Autodesk Inventor part; units mm, degrees
ref_plane "YZ Plane" through (0, 0, 0) normal (1, 0, 0) x (0, 1, 0)
ref_plane "XZ Plane" through (0, 0, 0) normal (0, 1, 0) x (-1, 0, 0)
ref_plane "XY Plane" through (0, 0, 0) normal (0, 0, 1) x (1, 0, 0)
sketch "Sketch1" plane through (0, 0, 0) normal (0, 0, 1) x (1, 0, 0)
  line L0 (0, 0) -> (0, 60)
  line L1 (0, 60) -> (80, 60)
  line L2 (80, 60) -> (80, 170)
  line L3 (80, 170) -> (280, 170)
  line L4 (280, 170) -> (280, 0)
  line L5 (0, 0) -> (35, 0)
  line L6 (35, 0) -> (35, 20)
  arc A0 (75, 20) -> (35, 20) centre (55, 20) ccw
  line L7 (75, 20) -> (75, 0)
  line L8 (140, 0) -> (140, 170) construction
  line L9 (75, 0) -> (140, 0)
  line L10 (280, 0) -> (245, 0)
  line L11 (245, 0) -> (245, 20)
  arc A1 (245, 20) -> (205, 20) centre (225, 20) ccw
  line L12 (205, 20) -> (205, 0)
  line L13 (205, 0) -> (140, 0)
  line L14 (145, 170) -> (215, 170)
  line L15 (215, 170) -> (215, 175)
  line L16 (215, 175) -> (145, 175)
  line L17 (145, 175) -> (145, 170)
  line L18 (280, 80) -> (275, 80)
  line L19 (275, 80) -> (275, 130)
  line L20 (275, 130) -> (280, 130)
  line L21 (280, 130) -> (280, 80)
  line L22 (10, 20) -> (15, 20)
  line L23 (15, 20) -> (15, 60)
  line L24 (15, 60) -> (10, 60)
  line L25 (10, 60) -> (10, 20)
  line L26 (20, 60) -> (60, 60)
  line L27 (60, 60) -> (60, 65)
  line L28 (60, 65) -> (20, 65)
  line L29 (20, 65) -> (20, 60)
  line L30 (160, 0) -> (160, -5)
  line L31 (160, -5) -> (120, -5)
  line L32 (120, -5) -> (120, 0)
  dimension "d0" = 60
  dimension "d2" = 110
  dimension "d5" = 20
  dimension "d6" = 40
  dimension "d7" = 70
  dimension "d8" = 5
  dimension "d9" = 5
  dimension "d10" = 50
  dimension "d13" = 5
  dimension "d14" = 40
  dimension "d17" = 40
  dimension "d18" = 5
  dimension "d19" = 40
  dimension "d20" = 5
  dimension "d21" = 20
  dimension "d22" = 0
  dimension "d23" = 170
  dimension "d27" = 35
  dimension "d28" = 80
extrude "Extrusion1" add sketch "Sketch1" along normal blind 5 contours L0 L1 L25 L22 L23 L2 L3 L4 L20 L19 L18 L10 L11 A1 L12 L13 L9 L7 A0 L6 L5 | L1 L23 L22 L25 | L29 L28 L27 L1 | L9 L13 L30 L31 L32 | L17 L16 L15 L3
sketch "Sketch2" plane through (0, 0, 5) normal (0, 0, 1) x (1, 0, 0)
  line L0 (215, 175) -> (145, 175)
  line L1 (145, 175) -> (145, 170)
  line L2 (120, -5) -> (160, -5)
  line L3 (160, -5) -> (160, 0)
  line L4 (0, 60) -> (0, 0)
  line L5 (20, 60) -> (0, 60)
  point P0 (175, 155)
  point P1 (185, 155)
  point P2 (135, 15)
  point P3 (145, 15)
  point P4 (20, 35)
  point P5 (20, 25)
  dimension "d43" = 10
  dimension "d44" = 20
  dimension "d45" = 20
  dimension "d46" = 30
  dimension "d47" = 20
  dimension "d48" = 20
  dimension "d49" = 10
  dimension "d50" = 15
  dimension "d51" = 10
  dimension "d52" = 20
  dimension "d53" = 20
  dimension "d54" = 25
hole "Hole1" at (175, 155, 5) at (185, 155, 5) at (135, 15, 5) at (145, 15, 5) at (20, 35, 5) at (20, 25, 5) direction (0, 0, -1) diameter 4 end through all
sketch "Sketch4" plane through (0, 0, 5) normal (0, 0, 1) x (1, 0, 0)
  line L0 (80, 170) -> (80, 60)
  line L1 (80, 60) -> (60, 60)
  point P0 (0, 0)
  point P1 (95, 80)
  point P2 (95, 90)
  dimension "d63" = 15
  dimension "d64" = 15
  dimension "d65" = 10
  dimension "d66" = 20
hole "Hole3" at (95, 80, 5) at (95, 90, 5) direction (0, 0, -1) diameter 4 end through all
properties part number "side"
Model file for the job. Use its own axes, mm. A direction names the side the tool comes from. Coordinates: 2 decimals unless noted, no trailing zeros. Loops run counter-clockwise (first coordinate to the right, second up) from the corner with the lowest first, then second, coordinate; pieces in that order, holes last. Notation, with made-up numbers: (62.25, -32) -> (72.25, -32) arc R4 cw to (72.25, -25) -> close; hole circle Ø2 at (16, 31.5). An arc over 180 degrees is marked (long way). Use one line per item in the form item = value. Start each with the question number.
(1) Cut at B-B on z = 3.1. Give the number of separate pieces and of enclosed holes in the cut face, and give its area (3 significant figures).
(2) Pull direction X, two halves, no side cores. Call faces 4 (the flat face through (10, 60, 2)), 5 (the flat face through (35, 10, 2)), 6 (the flat face through (20, 63, 2)): pulls with the +X half, pulls with the -X half, needs draft (parallel to the pull), parting line crosses it, or undercut.
(3) Cut at A-A on y = 140.5. Give the cut face in (x, z), and give its area (3 significant figures).
(4) Cut at C-C on x = 109. Give the cut face in (y, z).
(5) Tool access for faces 1 (the flat face through (70, 60, 2)), 2 (the flat face through (40, 65, 2)), 3 (the flat face through (205, 10, 2)): list every direction of +Z, -Z, +X, -X, +Y, -Y with a clear straight run to the whole face (end or side of a thin tool).
(6) Flat gauge pins, fed straight in: pin 1 (2.5 mm diameter, centred on x = 175, y = 155, fed in from +Z); pin 2 (2.5 mm diameter, centred on x = 121, z = 2, fed in from +Y); pin 3 (1.5 mm diameter, centred on x = 65.5, z = 3.5, fed in from +Y); pin 4 (3 mm diameter, centred on y = 124, z = 2, fed in from -X). Where does each tip first touch, or does it go through?
(7) Probe probe 1 along X at (y, z) = (155, 2); probe 2 along X at (y, z) = (15, 2.1); probe 3 along Y at (x, z) = (20.5, 2.6). List the from-to ranges inside material, lowest first. Write a range as from..to.
Values:
q1.separate_pieces = 1
q1.enclosed_holes = 8
q1.area = 36,300 mm2
q2.face_4 = needs draft
q2.face_5 = undercut
q2.face_6 = pulls with the -X half
q3.outline = (80, 0) -> (280, 0) -> (280, 5) -> (80, 5) -> close
q3.area = 1,000 mm2
q4.outline = (0, 0) -> (170, 0) -> (170, 5) -> (0, 5) -> close
q5.face_1 = +Z, -Z, +Y
q5.face_2 = +Z, -Z, -X, +Y
q5.face_3 = +Z, -Z, -Y
q6.pin_1 = through
q6.pin_2 = 170
q6.pin_3 = 60
q6.pin_4 = 80
q7.probe_1 = 80..173, 177..183, 187..280
q7.probe_2 = 0..35, 75..133, 137..143, 147..205, 245..280
q7.probe_3 = 0..23.06, 26.94..33.06, 36.94..65
